Read the model definition and answer for the solid it produces. Units are mm, in the model's axes. A direction names the side the tool comes from. Give positions to 0.01 mm unless a question says otherwise; leave off trailing zeros. Write each loop counter-clockwise with the first axis right and the second up, starting at its lowest first coordinate (ties: lowest second). Pieces come first, ordered by that corner, then holes. Notation, with made-up numbers: (-28, -28.75) -> (26, -28.75) arc R30 cw to (26, 5.25) -> close; hole circle Ø4 at (57, 69.5). An arc over 180 degrees is marked (long way). Write item = value, one per line.
from build123d import *

# Parameters (mm, degrees)
F1_DEPTH      = 36.6
F3_DEPTH      = 14.9
F3_DEPTH_BACK = 51.5
F4_R          = 5
F5_DEPTH      = 32.001
F6_T4_DEPTH   = 18.3
F6_S5_R       = 5
F6_T6_DEPTH   = 11
F6_T10_DEPTH  = 18.3
F6_S11_R      = 5
F6_T12_DEPTH  = 11
F6_T16_DEPTH  = 18.3
F6_S17_R      = 5
F6_T18_DEPTH  = 11
F6_T22_DEPTH  = 18.3
F6_S23_R      = 5
F6_T24_DEPTH  = 11
F6_T25_DEPTH  = 48.1
F6_T27_DEPTH  = 22.1993140666
F6_T29_DEPTH  = 22.1993140666
F6_T31_DEPTH  = 20.65
F6_T33_DEPTH  = 20.65


# Not quite as in the source:
# - a fillet or chamfer that OpenCascade refuses, or shapes differently, is made with other operations: its cross-section is extruded or revolved along the edge and cut away or added


with BuildPart() as f1:
    # F0 (on Front) → F1 (new body)
    with BuildSketch(Plane.XZ):
        Polygon((-28.4127721637, 8.7557665049), (-43.9127721637, 8.7557665049), (-43.9127721637, -1.2442334951), (-39.9127721637, -1.2442334951), (-32.4127721637, -23.2442334951), (-28.4127721637, -23.2442334951), align=None)
        Polygon((30.5872278363, 8.7557665049), (-28.4127721637, 8.7557665049), (-28.4127721637, -23.2442334951), (-12.9127721637, -23.2442334951), (-12.9127721637, -9.2442334951), (15.0872278363, -9.2442334951), (15.0872278363, -23.2442334951), (30.5872278363, -23.2442334951), align=None)
        Polygon((46.0872278363, 8.7557665049), (30.5872278363, 8.7557665049), (30.5872278363, -23.2442334951), (34.5872278363, -23.2442334951), (42.0872278363, -1.2442334951), (46.0872278363, -1.2442334951), align=None)
    extrude(amount=F1_DEPTH)

    # F2 (on face) → F3 (join, two sides)
    with BuildSketch(Plane(origin=(0, 0, 0), x_dir=(-1, 0, 0), z_dir=(0, 1, 0))) as f3_sk:
        Polygon((28.4127721637, 8.7557665049), (-30.5872278363, 8.7557665049), (-30.5872278363, -23.2442334951), (-15.0872278363, -23.2442334951), (-15.0872278363, -9.2442334951), (12.9127721637, -9.2442334951), (12.9127721637, -23.2442334951), (28.4127721637, -23.2442334951), align=None)
    extrude(amount=F3_DEPTH)
    extrude(f3_sk.sketch, amount=-F3_DEPTH_BACK)

    # F4 (on face) → F5 (cut, through all)
    with BuildSketch(Plane.XY.offset(8.7557665049)):
        with Locations((-34.9127721637, -18.3)):
            Circle(F4_R)
        with Locations((37.0872278363, -18.3)):
            Circle(F4_R)
    extrude(amount=-F5_DEPTH, mode=Mode.SUBTRACT)

    # F6: fillet of radius 2.3 on 20 edges, made by hand


with BuildPart() as f6_tool2:
    # F6_s3 → F6_t4 (new body)
    with BuildSketch(Plane.XZ.offset(18.3)):
        with BuildLine():
            ThreePointArc((-41.5586603808, -1.2442334951), (-40.2201808476, -1.6738130774), (-39.381686948, -2.8020834612))
            Line((-39.381686948, -2.8020834612), (-39.9127721637, -1.2442334951))
            Line((-39.9127721637, -1.2442334951), (-41.5586603808, -1.2442334951))
        make_face()
    extrude(amount=F6_T4_DEPTH)

    # F6_s5 → F6_t6 (cut, symmetric)
    with BuildSketch(Plane.XY.offset(-2)):
        with Locations((-34.9127721637, -18.3)):
            Circle(F6_S5_R)
    extrude(amount=F6_T6_DEPTH, both=True, mode=Mode.SUBTRACT)


with BuildPart() as f1_1:
    add(f1.part)

    # F6_t1: union F6_tool2
    add(f6_tool2.part)


with BuildPart() as f6_tool8:
    # F6_s9 → F6_t10 (new body)
    with BuildSketch(Plane.XZ.offset(18.3)):
        with BuildLine():
            ThreePointArc((43.7331160534, -1.2442334951), (42.3946365201, -1.6738130774), (41.5561426205, -2.8020834612))
            Line((41.5561426205, -2.8020834612), (42.0872278363, -1.2442334951))
            Line((42.0872278363, -1.2442334951), (43.7331160534, -1.2442334951))
        make_face()
    extrude(amount=F6_T10_DEPTH)

    # F6_s11 → F6_t12 (cut, symmetric)
    with BuildSketch(Plane.XY.offset(-2)):
        with Locations((37.0872278363, -18.3)):
            Circle(F6_S11_R)
    extrude(amount=F6_T12_DEPTH, both=True, mode=Mode.SUBTRACT)


with BuildPart() as f1_2:
    add(f1_1.part)

    # F6_t7: union F6_tool8
    add(f6_tool8.part)


with BuildPart() as f6_tool14:
    # F6_s15 → F6_t16 (new body)
    with BuildSketch(Plane.XZ):
        with BuildLine():
            ThreePointArc((43.7331160534, -1.2442334951), (42.3946365201, -1.6738130774), (41.5561426205, -2.8020834612))
            Line((41.5561426205, -2.8020834612), (42.0872278363, -1.2442334951))
            Line((42.0872278363, -1.2442334951), (43.7331160534, -1.2442334951))
        make_face()
    extrude(amount=F6_T16_DEPTH)

    # F6_s17 → F6_t18 (cut, symmetric)
    with BuildSketch(Plane.XY.offset(-2)):
        with Locations((37.0872278363, -18.3)):
            Circle(F6_S17_R)
    extrude(amount=F6_T18_DEPTH, both=True, mode=Mode.SUBTRACT)


with BuildPart() as f1_3:
    add(f1_2.part)

    # F6_t13: union F6_tool14
    add(f6_tool14.part)


with BuildPart() as f6_tool20:
    # F6_s21 → F6_t22 (new body)
    with BuildSketch(Plane.XZ):
        with BuildLine():
            ThreePointArc((-41.5586603808, -1.2442334951), (-40.2201808476, -1.6738130774), (-39.381686948, -2.8020834612))
            Line((-39.381686948, -2.8020834612), (-39.9127721637, -1.2442334951))
            Line((-39.9127721637, -1.2442334951), (-41.5586603808, -1.2442334951))
        make_face()
    extrude(amount=F6_T22_DEPTH)

    # F6_s23 → F6_t24 (cut, symmetric)
    with BuildSketch(Plane.XY.offset(-2)):
        with Locations((-34.9127721637, -18.3)):
            Circle(F6_S23_R)
    extrude(amount=F6_T24_DEPTH, both=True, mode=Mode.SUBTRACT)


with BuildPart() as f1_4:
    add(f1_3.part)

    # F6_t19: union F6_tool20
    add(f6_tool20.part)

    # F6_s26 → F6_t25 (cut)
    with BuildSketch(Plane.XZ.offset(-5.75)):
        with BuildLine():
            ThreePointArc((-43.9127721637, 1.0557665049), (-43.2391177605, -0.5705790919), (-41.6127721637, -1.2442334951))
            Line((-41.6127721637, -1.2442334951), (-43.9127721637, -1.2442334951))
            Line((-43.9127721637, -1.2442334951), (-43.9127721637, 1.0557665049))
        make_face()
        with BuildLine():
            ThreePointArc((-43.9127721637, 6.4557665049), (-43.2391177605, 8.0821121016), (-41.6127721637, 8.7557665049))
            Line((-41.6127721637, 8.7557665049), (-43.9127721637, 8.7557665049))
            Line((-43.9127721637, 8.7557665049), (-43.9127721637, 6.4557665049))
        make_face()
        with BuildLine():
            ThreePointArc((46.0872278363, 6.4557665049), (45.413573433, 8.0821121016), (43.7872278363, 8.7557665049))
            Line((43.7872278363, 8.7557665049), (46.0872278363, 8.7557665049))
            Line((46.0872278363, 8.7557665049), (46.0872278363, 6.4557665049))
        make_face()
        with BuildLine():
            ThreePointArc((46.0872278363, 1.0557665049), (45.413573433, -0.5705790919), (43.7872278363, -1.2442334951))
            Line((43.7872278363, -1.2442334951), (46.0872278363, -1.2442334951))
            Line((46.0872278363, -1.2442334951), (46.0872278363, 1.0557665049))
        make_face()
    extrude(amount=F6_T25_DEPTH, mode=Mode.SUBTRACT)

    # F6_s28 → F6_t27 (cut)
    with BuildSketch(Plane.XZ.offset(18.5154064762)):
        with BuildLine():
            ThreePointArc((-30.7668839466, -23.2442334951), (-32.1053634799, -22.8146539129), (-32.9438573795, -21.6863835291))
            Line((-32.9438573795, -21.6863835291), (-32.4127721637, -23.2442334951))
            Line((-32.4127721637, -23.2442334951), (-30.7668839466, -23.2442334951))
        make_face()
        with BuildLine():
            ThreePointArc((35.118313052, -21.6863835291), (34.2798191524, -22.8146539129), (32.9413396192, -23.2442334951))
            Line((32.9413396192, -23.2442334951), (34.5872278363, -23.2442334951))
            Line((34.5872278363, -23.2442334951), (35.118313052, -21.6863835291))
        make_face()
    extrude(amount=F6_T27_DEPTH, mode=Mode.SUBTRACT)

    # F6_s30 → F6_t29 (cut)
    with BuildSketch(Plane.XZ.offset(-4.1147205427)):
        with BuildLine():
            ThreePointArc((-30.7668839466, -23.2442334951), (-32.1053634799, -22.8146539129), (-32.9438573795, -21.6863835291))
            Line((-32.9438573795, -21.6863835291), (-32.4127721637, -23.2442334951))
            Line((-32.4127721637, -23.2442334951), (-30.7668839466, -23.2442334951))
        make_face()
        with BuildLine():
            ThreePointArc((35.118313052, -21.6863835291), (34.2798191524, -22.8146539129), (32.9413396192, -23.2442334951))
            Line((32.9413396192, -23.2442334951), (34.5872278363, -23.2442334951))
            Line((34.5872278363, -23.2442334951), (35.118313052, -21.6863835291))
        make_face()
    extrude(amount=F6_T29_DEPTH, mode=Mode.SUBTRACT)

    # F6_s32 → F6_t31 (cut)
    with BuildSketch(Plane.XZ.offset(36.6)):
        with BuildLine():
            ThreePointArc((-28.4127721637, -20.9442334951), (-27.7391177605, -22.5705790919), (-26.1127721637, -23.2442334951))
            Line((-26.1127721637, -23.2442334951), (-28.4127721637, -23.2442334951))
            Line((-28.4127721637, -23.2442334951), (-28.4127721637, -20.9442334951))
        make_face()
        with BuildLine():
            ThreePointArc((-28.4127721637, 6.4557665049), (-27.7391177605, 8.0821121016), (-26.1127721637, 8.7557665049))
            Line((-26.1127721637, 8.7557665049), (-28.4127721637, 8.7557665049))
            Line((-28.4127721637, 8.7557665049), (-28.4127721637, 6.4557665049))
        make_face()
        with BuildLine():
            ThreePointArc((30.5872278363, 6.4557665049), (29.913573433, 8.0821121016), (28.2872278363, 8.7557665049))
            Line((28.2872278363, 8.7557665049), (30.5872278363, 8.7557665049))
            Line((30.5872278363, 8.7557665049), (30.5872278363, 6.4557665049))
        make_face()
        with BuildLine():
            ThreePointArc((28.2872278363, -23.2442334951), (29.913573433, -22.5705790919), (30.5872278363, -20.9442334951))
            Line((30.5872278363, -20.9442334951), (30.5872278363, -23.2442334951))
            Line((30.5872278363, -23.2442334951), (28.2872278363, -23.2442334951))
        make_face()
    extrude(amount=F6_T31_DEPTH, mode=Mode.SUBTRACT)

    # F6_s34 → F6_t33 (cut)
    with BuildSketch(Plane.XZ.offset(-20.65)):
        with BuildLine():
            ThreePointArc((-28.4127721637, -20.9442334951), (-27.7391177605, -22.5705790919), (-26.1127721637, -23.2442334951))
            Line((-26.1127721637, -23.2442334951), (-28.4127721637, -23.2442334951))
            Line((-28.4127721637, -23.2442334951), (-28.4127721637, -20.9442334951))
        make_face()
        with BuildLine():
            ThreePointArc((-28.4127721637, 6.4557665049), (-27.7391177605, 8.0821121016), (-26.1127721637, 8.7557665049))
            Line((-26.1127721637, 8.7557665049), (-28.4127721637, 8.7557665049))
            Line((-28.4127721637, 8.7557665049), (-28.4127721637, 6.4557665049))
        make_face()
        with BuildLine():
            ThreePointArc((30.5872278363, 6.4557665049), (29.913573433, 8.0821121016), (28.2872278363, 8.7557665049))
            Line((28.2872278363, 8.7557665049), (30.5872278363, 8.7557665049))
            Line((30.5872278363, 8.7557665049), (30.5872278363, 6.4557665049))
        make_face()
        with BuildLine():
            ThreePointArc((30.5872278363, -20.9442334951), (29.913573433, -22.5705790919), (28.2872278363, -23.2442334951))
            Line((28.2872278363, -23.2442334951), (30.5872278363, -23.2442334951))
            Line((30.5872278363, -23.2442334951), (30.5872278363, -20.9442334951))
        make_face()
    extrude(amount=F6_T33_DEPTH, mode=Mode.SUBTRACT)


solid = f1_4.part
(1) The part is cut by section D-D on x = 1. Determine the outline of the cut face in (y, z).
Checks:
outline = (-51.5, -9.24) -> (14.9, -9.24) -> (14.9, 8.76) -> (-51.5, 8.76) -> close
(2) The part is cut by section A-A on z = -17. Determine the outline of the cut face in (x, y), plus the area to 3 significant figures.
Checks:
outline = (-34.54, -36.6) -> (-28.41, -36.6) -> (-28.41, -51.5) -> (-12.91, -51.5) -> (-12.91, 14.9) -> (-28.41, 14.9) -> (-28.41, 0) -> (-34.54, 0) -> (-34.54, -13.31) arc R5 cw to (-34.54, -23.29) -> close; (15.09, -51.5) -> (30.59, -51.5) -> (30.59, -36.6) -> (36.72, -36.6) -> (36.72, -23.29) arc R5 cw to (36.72, -13.31) -> (36.72, 0) -> (30.59, 0) -> (30.59, 14.9) -> (15.09, 14.9) -> close
area = 2,440 mm²
(3) The part is cut by section C-C on y = -3. Determine the outline of the cut face in (x, z).
Checks:
outline = (-43.91, 1.06) arc R2.3 ccw to (-41.61, -1.24) -> (-41.56, -1.24) arc R2.3 cw to (-39.38, -2.8) -> (-32.94, -21.69) arc R2.3 ccw to (-30.77, -23.24) -> (-12.91, -23.24) -> (-12.91, -9.24) -> (15.09, -9.24) -> (15.09, -23.24) -> (32.94, -23.24) arc R2.3 ccw to (35.12, -21.69) -> (41.56, -2.8) arc R2.3 cw to (43.73, -1.24) -> (43.79, -1.24) arc R2.3 ccw to (46.09, 1.06) -> (46.09, 6.46) arc R2.3 ccw to (43.79, 8.76) -> (-41.61, 8.76) arc R2.3 ccw to (-43.91, 6.46) -> close
(4) Given P1, Ø1, axis at y = -19, z = -13.5, coming from the +X side; P2, Ø15.5, axis at y = -24, z = -18.5, coming from the +X side; P3, Ø4.5, axis at y = -41.5, z = -12.5, coming from the -X side; P4, Ø9, axis at x = 37.09, y = -18.3, coming from the -Z side, each flat-ended and moving along its own axis, determine where each tip first touches the part or whether it passes through.
Checks:
P1 = 32.23
P2 = 38.85
P3 = -28.41
P4 = through
(5) A tool of negligible diameter and unlimited length cuts with its end or side. For faces 4 (the cylindrical face through (29.931, -43.946, 8.064)), 5 (the cylindrical face through (29.931, 7.554, 8.064)), 6 (the flat face through (30.587, -44, -7)), from which of +Z, -Z, +X, -X, +Y, -Y can it reach the whole face along a straight path? Write none if from no direction.
Checks:
face_4 = +Z, +X, -Y
face_5 = +Z, +X, +Y
face_6 = +Z, -Z, +X, -Y
(6) The part is cut by section B-B on y = -18.3. Determine the outline of the cut face in (x, z), plus the area to 3 significant figures.
Checks:
outline = (-43.91, 1.06) arc R2.3 ccw to (-41.61, -1.24) -> (-41.56, -1.24) arc R2.3 cw to (-39.91, -1.94) -> (-39.91, 8.76) -> (-41.61, 8.76) arc R2.3 ccw to (-43.91, 6.46) -> close; (-29.91, -23.24) -> (-12.91, -23.24) -> (-12.91, -9.24) -> (15.09, -9.24) -> (15.09, -23.24) -> (32.09, -23.24) -> (32.09, 8.76) -> (-29.91, 8.76) -> close; (42.09, -1.94) arc R2.3 cw to (43.73, -1.24) -> (43.79, -1.24) arc R2.3 ccw to (46.09, 1.06) -> (46.09, 6.46) arc R2.3 ccw to (43.79, 8.76) -> (42.09, 8.76) -> close
area = 1,670 mm²
(7) For a pull along X with two mould halves and no side action, classify faces 1 (the flat face through (-43.913, -18, 4)), 2 (the cylindrical face through (45.431, -18.044, 8.064)), 3 (the flat face through (15.087, -18, -16)) as released by +X, released by -X, zero draft, split by the parting line, or undercut.
Checks:
face_1 = released by -X
face_2 = released by +X
face_3 = undercut
(8) Consider L1, parallel to X at y = -47.5, z = -12; L2, parallel to X at y = -18, z = -15; L3, parallel to Z at x = 10, y = 7. Determine where each line is inside the solid, lowest interval first.
Checks:
L1 = -28.41 to -12.91, 15.09 to 30.59
L2 = -29.92 to -12.91, 15.09 to 32.1
L3 = -9.24 to 8.76
